Geometry: final body of the model. Coordinates: model frame, mm. A direction names the side the tool comes from. Round coordinates to 2 decimals unless told otherwise and drop trailing zeros. Loops run counter-clockwise (first coordinate to the right, second up) from the corner with the lowest first, then second, coordinate; pieces in that order, holes last. Notation, with made-up numbers: (-29, 48.5) - (5, 48.5) arc R12 cw to (5, 54.5) - close; hole circle Ø1 at (77.25, -12.5). An arc over 180 degrees is marked (long way). Use CSV: the item, a comma, the result in double quotes.
from build123d import *

# Parameters (mm, degrees)
F0_R     = 5
F0_R_2   = 4.25
F0_R_3   = 2.5
F1_DEPTH = 1
F2_DEPTH = 6
F3_START = 5
F3_DEPTH = 1


with BuildPart() as f1:
    # F0 (on Top) → F1 (new body)
    with BuildSketch(Plane.XY):
        Circle(F0_R)
        Circle(F0_R_2, mode=Mode.SUBTRACT)
        Circle(F0_R_2)
        Circle(F0_R_3, mode=Mode.SUBTRACT)
        Circle(F0_R_3)
    extrude(amount=F1_DEPTH)

    # F0 (on Top) → F2 (join)
    with BuildSketch(Plane.XY):
        Circle(F0_R)
        Circle(F0_R_2, mode=Mode.SUBTRACT)
    extrude(amount=F2_DEPTH)

    # F0 (on Top) → F3 (join)
    with BuildSketch(Plane.XY.offset(F3_START)):
        Circle(F0_R_2)
        Circle(F0_R_3, mode=Mode.SUBTRACT)
    extrude(amount=F3_DEPTH)


solid = f1.part
Item 1: Mould query, pull axis X, two halves, no side actions, for faces 1 (the flat face through (2, -2, 6)), 2 (the cylindrical face through (-1.08, -4.88, 2.96)), 3 (the cylindrical face through (-0.54, -2.44, 5.49)). Classes: released by +X, released by -X, zero draft, split by the parting line, or undercut.
Final values:
face 1,"zero draft"
face 2,"split by the parting line"
face 3,"undercut"
Item 2: Material intervals for line 1 (Y direction, x = 0, z = 5.3); line 2 (Z direction, x = 2.75, y = 0); line 3 (Y direction, x = 0, z = 3.9), sorted ascending.
Final values:
line 1,"y = -5 to -2.5, 2.5 to 5"
line 2,"z = 0 to 1, 5 to 6"
line 3,"y = -5 to -4.25, 4.25 to 5"
Item 3: Reachability of faces 4 (the flat face through (0, 0, 1)), 5 (the flat face through (0, 0, 0)) from +Z, -Z, +X, -X, +Y, -Y: full face, straight path, thin tool, end or side. Return the list, or none.
Final values:
face 4,"none"
face 5,"-Z, +X, -X, +Y, -Y"
Item 4: Section D-D on z = 3.4. Return the cut outline in (x, y).
Final values:
outline,"circle Ø10 at (0, 0); hole circle Ø8.5 at (0, 0)"
Item 5: Section C-C on x = -3.5. Return the cut outline in (y, z).
Final values:
outline,"(-3.57, 0) - (3.57, 0) - (3.57, 6) - (-3.57, 6) - close; hole (-2.41, 1) - (2.41, 1) - (2.41, 5) - (-2.41, 5) - close"
Item 6: Section A-A on y = 0. Return the cut outline in (x, z).
Final values:
outline,"(-5, 0) - (5, 0) - (5, 6) - (2.5, 6) - (2.5, 5) - (4.25, 5) - (4.25, 1) - (-4.25, 1) - (-4.25, 5) - (-2.5, 5) - (-2.5, 6) - (-5, 6) - close"
Item 7: Pin query (flat end, axial travel): P1, Ø1.5, axis at y = 2, z = 2, coming from the -X side; P2, Ø2, axis at x = -3.5, z = 4, coming from the +Y side. Return the tip coordinate at first contact, or that it passes through.
Final values:
P1,"stops at x = -4.84"
P2,"stops at y = 4.33"
